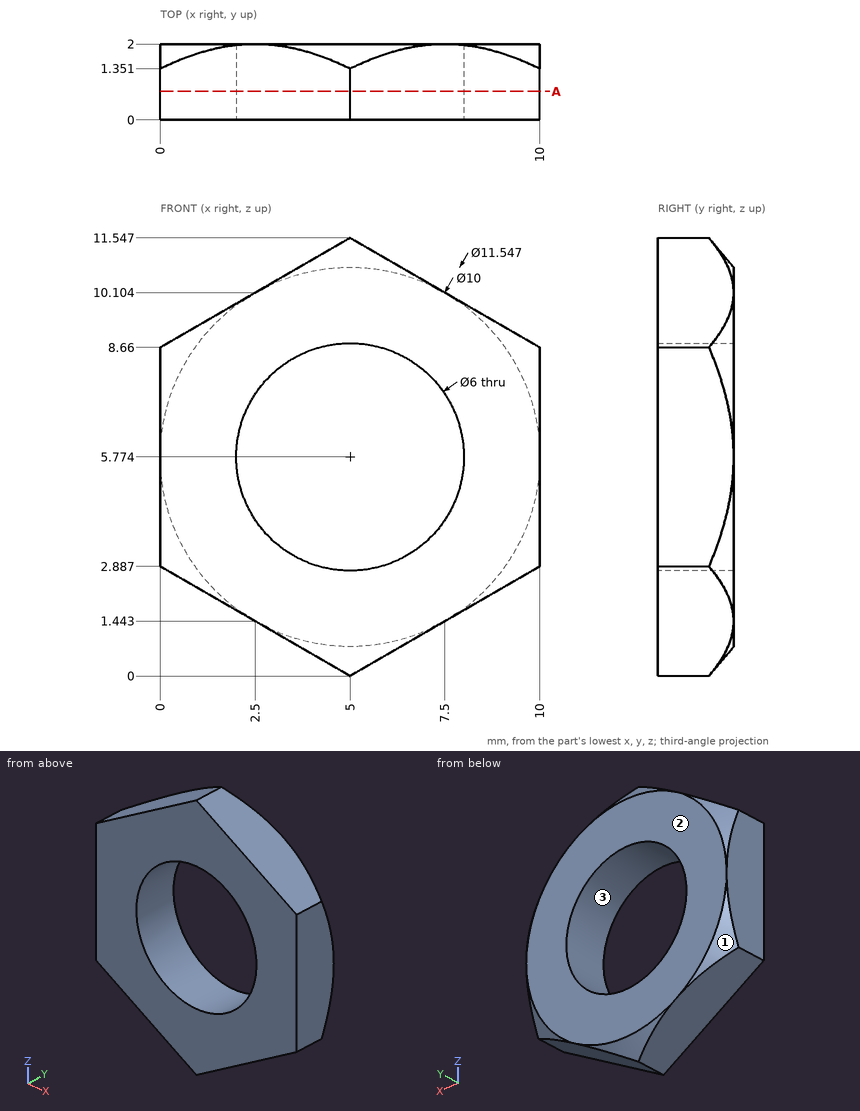
Geometry check sheet. Reference: drawing and pictorial views, mm from the part's lowest x, y, z. Round coordinates to 2 decimals unless told otherwise and drop trailing zeros. Order: outer loops, then holes, each group sorted by start corner. A loop starts at its lowest first (then second) coordinate and runs counter-clockwise, first axis right, second up. Notation, with made-up numbers: (52.25, -9) - (71.25, -9) arc R20 ccw to (71.25, 6) - close; hole circle Ø5 at (-32, 35.5). An arc over 180 degrees is marked (long way). Write item = value, one per line.
Q1. Thickness scan on line 1 along X through (y, z) = (1.7, 4); line 2 along Z through (x, y) = (4.75, 1.25) (1 decimal); line 3 along X through (y, z) = (1.95, 5.25) (1 decimal). Record the ranges inside material, lowest first.
Computed:
line_1 = 0 to 2.58, 7.42 to 10
line_2 = 0.1 to 2.8, 8.8 to 11.4
line_3 = 0 to 2, 8 to 10
Q2. Section check A-A (y = 0.75). Record the boundary of the cut face in (x, z).
Computed:
outline = (0, 2.89) - (5, 0) - (10, 2.89) - (10, 8.66) - (5, 11.55) - (0, 8.66) - close; hole circle Ø6 at (5, 5.77)
Q3. Go/stop test with a flat-tipped pin: pin 1 (1 mm diameter, centred on x = 5.5, z = 5, fed in from +Y). Record where the tip stops, or that it passes through.
Computed:
pin_1 = through
Q4. Draft check along Z on the marked faces 1, 2 and 3. Enter one of: pulls with the +Z half, pulls with the -Z half, needs draft (parallel to the pull), parting line crosses it, or undercut.
Computed:
face_1 = pulls with the -Z half
face_2 = needs draft
face_3 = undercut
